```python
from build123d import *

# Parameters (mm, degrees)
SKETCH2_R           = 25.0063
SKETCH2_R_2         = 11.9126
BOSS_EXTRUDE2_DEPTH = 20.0025
SKETCH2_3_R         = 7.9375
SKETCH2_3_R_2       = 5.9563
BOSS_EXTRUDE3_DEPTH = 12.4968
FILLET1_R           = 3.175


with BuildPart() as part:
    # Sketch2 → Boss-Extrude2 (new, symmetric)
    with BuildSketch(Plane(origin=(0, 0, 0), x_dir=(1, 0, 0), z_dir=(0, 1, 0))):
        with Locations(Location((0, 0, 0), (0, 0, 270))):
            Circle(SKETCH2_R)
        with Locations(Location((0, 0, 0), (0, 0, 270))):
            Circle(SKETCH2_R_2, mode=Mode.SUBTRACT)
    extrude(amount=BOSS_EXTRUDE2_DEPTH, both=True)

    # Sketch2<3> → Boss-Extrude3 (add, symmetric)
    with BuildSketch(Plane(origin=(0, 0, 0), x_dir=(1, 0, 0), z_dir=(0, 1, 0))):
        with BuildLine():
            ThreePointArc((-14.627829046, -20.281559533), (-18.962185595, 16.301857476), (17.857447567, 17.505045161))
            ThreePointArc((17.857447567, 17.505045161), (10.712225835, 35.0012), (17.857447567, 52.497354839))
            ThreePointArc((17.857447567, 52.497354839), (12.561079617, 91.624941907), (-24.05225317, 76.843756383))
            ThreePointArc((-24.05225317, 76.843756383), (-42.87857023, 47.021182923), (-74.850980968, 32.135584063))
            ThreePointArc((-74.850980968, 32.135584063), (-98.995210512, -14.684053906), (-46.965085328, -22.923495222))
            ThreePointArc((-46.965085328, -22.923495222), (-31.283411202, -15.642216981), (-14.627829046, -20.281559533))
        make_face()
        with Locations(Location((-70.0024, 0, 0), (0, 0, 270))):
            Circle(SKETCH2_3_R, mode=Mode.SUBTRACT)
        with Locations(Location((0, 70.0024, 0), (0, 0, 270))):
            Circle(SKETCH2_3_R_2, mode=Mode.SUBTRACT)
    extrude(amount=BOSS_EXTRUDE3_DEPTH, both=True)

    # Fillet1
    # the kernel refuses this fillet: 3.175 mm, written as the material it takes off along each edge
    with BuildSketch(Plane(origin=(-84.17677836, 12.4968, -93.945410073), x_dir=(0.9618477411525731, 0, 0.2735853118127743), z_dir=(0.2735853118127743, 0, -0.9618477411525731))) as fillet1_piece_1:
        with BuildLine():
            CenterArc((62.5094 + FILLET1_R, FILLET1_R), FILLET1_R, 180, 90)
            Line((62.5094, FILLET1_R), (62.5094, 0))
            Line((62.5094, 0), (62.5094 + FILLET1_R, 0))
        make_face()
    revolve(axis=Axis((-84.17677836, 12.4968, -93.945410073), (0, -1, 0)), revolution_arc=65.542266938, mode=Mode.SUBTRACT)
    with BuildSketch(Plane(origin=(-29.248229028, 12.4968, 40.552818629), x_dir=(-0.7088557190961631, 0, -0.705353506764276), z_dir=(-0.705353506764276, 0, 0.7088557190961631))) as fillet1_piece_2_section:
        with BuildLine():
            CenterArc((24.9936 + FILLET1_R, FILLET1_R), FILLET1_R, 180, 90)
            Line((24.9936 + FILLET1_R, 0), (24.9936, 0))
            Line((24.9936, 0), (24.9936, FILLET1_R))
        make_face()
    fillet1_piece_2 = revolve(axis=Axis((-29.248229028, 12.4968, 40.552818629), (0, -1, 0)), revolution_arc=99.144440238, mode=Mode.PRIVATE)
    fillet1_piece_2 = fillet1_piece_2 - Plane(origin=(0, 11.594758581, 0), x_dir=(0, 0, 1), z_dir=(0, 1, 0)) * Cylinder(25.0063, 113, mode=Mode.PRIVATE)
    add(fillet1_piece_2, mode=Mode.SUBTRACT)
    with BuildSketch(Plane(origin=(35.705825835, 12.4968, -35.0012), x_dir=(-0.45970021745025064, 0, 0.8880741579824245), z_dir=(0.8880741579824245, 0, 0.45970021745025064))) as fillet1_piece_3_section:
        with BuildLine():
            CenterArc((24.9936 + FILLET1_R, FILLET1_R), FILLET1_R, 180, 90)
            Line((24.9936, FILLET1_R), (24.9936, 0))
            Line((24.9936, 0), (24.9936 + FILLET1_R, 0))
        make_face()
    fillet1_piece_3 = revolve(axis=Axis((35.705825835, 12.4968, -35.0012), (0, -1, 0)), revolution_arc=107.06127711, mode=Mode.PRIVATE)
    fillet1_piece_3 = fillet1_piece_3 - Plane(origin=(0, 11.595953035, 0), x_dir=(0, 0, 1), z_dir=(0, 1, 0)) * Cylinder(25.0063, 113, mode=Mode.PRIVATE)
    add(fillet1_piece_3, mode=Mode.SUBTRACT)
    with BuildSketch(Plane(origin=(-70.0024, 12.4968, 0), x_dir=(-0.1491903200484399, 0, -0.9888084993586191), z_dir=(0.9888084993586191, 0, -0.1491903200484399))) as fillet1_piece_4:
        with BuildLine():
            CenterArc((32.4993 - FILLET1_R, -FILLET1_R), FILLET1_R, 0, 90)
            Line((32.4993, -FILLET1_R), (32.4993, 0))
            Line((32.4993, 0), (32.4993 - FILLET1_R, 0))
        make_face()
    revolve(axis=Axis((-70.0024, 12.4968, 0), (0, 1, 0)), revolution_arc=216.561882249, mode=Mode.SUBTRACT)
    with BuildSketch(Plane(origin=(0, 12.4968, -70.0024), x_dir=(0.7141179449388714, 0, 0.7000254000508005), z_dir=(-0.7000254000508005, 0, 0.7141179449388714))) as fillet1_piece_5:
        with BuildLine():
            CenterArc((25.0063 - FILLET1_R, -FILLET1_R), FILLET1_R, 0, 90)
            Line((25.0063, -FILLET1_R), (25.0063, 0))
            Line((25.0063, 0), (25.0063 - FILLET1_R, 0))
        make_face()
    revolve(axis=Axis((0, 12.4968, -70.0024), (0, 1, 0)), revolution_arc=208.551316171, mode=Mode.SUBTRACT)


solid = part.part
```
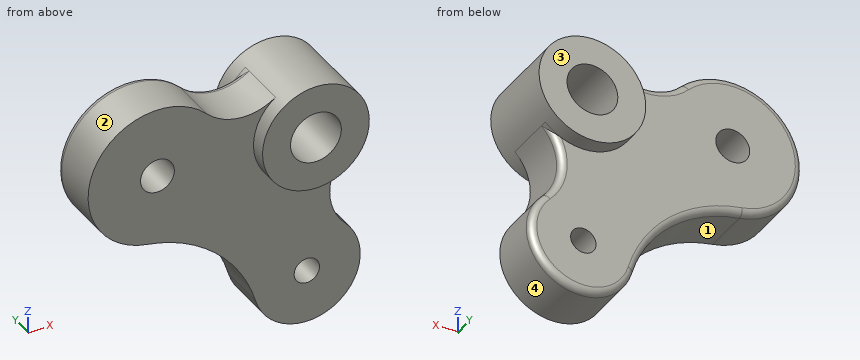
Geometry check sheet. Reference: the model listing, model coordinates, mm. Face numbers are marked on the shaded views. Round coordinates to 2 decimals unless told otherwise and drop trailing zeros. Order: outer loops, then holes, each group sorted by start corner. A loop starts at its lowest first (then second) coordinate and runs counter-clockwise, first axis right, second up. Notation, with made-up numbers: M -36.75,-27 L 0.25,-27 A25 cw 0.25,-12 Z; hole C 13.5,-29 d1. An arc over 180 degrees is marked long. Write item = value, one per line.
Q1. Section check A-A (x = 0). Give the number of separate pieces and of enclosed holes in the cut face, plus the area to 3 significant figures.
Answer block:
separate_pieces = 3
enclosed_holes = 0
area = 2,500 mm^2
Q2. Scan lines: line 1 (X direction, y = 6, z = 0); line 2 (X direction, y = 11, z = 0); line 3 (Y direction, x = -45, z = -23). Record each from-to range of solid material in increasing order.
Answer block:
line_1 = -102.5 to -77.94, -62.06 to -11.91, 11.91 to 25.01
line_2 = -102.02 to -77.94, -62.06 to -11.91, 11.91 to 25.01
line_3 = -12.5 to 12.5
Q3. Depth check by flat-ended pin: pin 1 Ø4 at (x, z) = (-70.5, -13) entering from -Y; pin 2 Ø6 at (y, z) = (11, 1.5) entering from +X; pin 3 Ø3 at (x, y) = (-66, -12) entering from -Z; pin 4 Ø21.5 at (x, z) = (0, 0) entering from -Y. Enter the tip coordinate at first touch or a pass-through.
Answer block:
pin_1 = -12.5
pin_2 = 25.01
pin_3 = -34.61
pin_4 = through
Q4. Section check D-D (y = -17). Enter the section's corners in (x, z).
Answer block:
outline = C 0,0 d50.01; hole C 0,0 d23.83
Q5. Section check C-C (y = -5.5). Enter the section's corners in (x, z) (1 decimal), plus the area to 3 significant figures.
Answer block:
outline = M -74.9,-32.1 A62.5 cw -24.1,-76.8 A25 ccw long 17.9,-52.5 A25 cw 17.9,-17.5 A25 ccw -14.6,20.3 A25 cw -47,22.9 A32.5 ccw long Z; hole C -70,0 d15.9; hole C 0,0 d23.8; hole C 0,-70 d11.9
area = 9,050 mm^2
Q6. Release check for a two-part mould opening along Z. For the marked faces 1, 2, 3 and 4 record: released by +Z, released by -Z, zero draft, split by the parting line, or undercut.
Answer block:
face_1 = released by -Z
face_2 = split by the parting line
face_3 = zero draft
face_4 = undercut
